For this review, take the finished solid that the model builds, in its own axes (mm). Coordinates: 2 decimals unless noted, no trailing zeros. Loops run counter-clockwise (first coordinate to the right, second up) from the corner with the lowest first, then second, coordinate; pieces in that order, holes last.
1. Take a section at B-B, the plane y = 2.2. Count the separate pieces of the cut face and the enclosed holes in it, then the cut area to 3 significant figures.
2. Take a section at C-C, the plane x = 0. State the section outline as (y, z) points.
3. Clearance check with flat-ended pins moving along their axes: P1, Ø3, axis at y = 4.5, z = -13, coming from the +X side; P2, Ø1, axis at y = 4, z = -2.5, coming from the +X side. State where each tip first meets the part, or that it passes through.
4. Mouldability with a two-part tool opening along Z and no side actions: class faces 1 (the face through (195.482, 2.535, -17.871)), 2 (the face through (-195.871, 2.535, 17.482)), 3 (the face through (-179.045, 2.465, -1.409)) as pulls with the +Z half, pulls with the -Z half, needs draft (parallel to the pull), parting line crosses it, or undercut.
5. To check wall thickness, follow probe 1 along X at (y, z) = (1, 0); probe 2 along Z at (x, y) = (163, 0.35); probe 3 along X at (y, z) = (2.05, -9.5). State the ranges of each line that lie inside material, in increasing order.
6. Take a section at A-A, the plane x = 172.7. State the section outline as (y, z) points.
```python
from build123d import *

# Parameters (mm, degrees)
SKETCH_1_W      = 406
SKETCH_1_H      = 50
SKETCH_1_R      = 6.5
SKETCH_1_R_2    = 9
SKETCH_1_R_3    = 2
EXTRUDE_1_DEPTH = 5
FILLET_1_R      = 25


with BuildPart() as part:
    # ｽｹｯﾁ1 → ﾎﾞｽ - 押し出し1 (new body)
    with BuildSketch(Plane(origin=(0, 0, 0), x_dir=(1, 0, 0), z_dir=(0, 1, 0))):
        Rectangle(SKETCH_1_W, SKETCH_1_H)
        with Locations(Location((172.7, 0, 0), (0, 0, 270))):
            Circle(SKETCH_1_R, mode=Mode.SUBTRACT)
        with Locations(Location((-172.7, 0, 0), (0, 0, 270))):
            Circle(SKETCH_1_R, mode=Mode.SUBTRACT)
        with Locations(Location((0, 0, 0), (0, 0, 270))):
            Circle(SKETCH_1_R_2, mode=Mode.SUBTRACT)
        with Locations(Location((12.02081528, 12.02081528, 0), (0, 0, 270))):
            Circle(SKETCH_1_R_3, mode=Mode.SUBTRACT)
        with Locations(Location((12.02081528, -12.02081528, 0), (0, 0, 270))):
            Circle(SKETCH_1_R_3, mode=Mode.SUBTRACT)
        with Locations(Location((-182.953048327, 10.253048327, 0), (0, 0, 270))):
            Circle(SKETCH_1_R_3, mode=Mode.SUBTRACT)
        with Locations(Location((182.953048327, 10.253048327, 0), (0, 0, 270))):
            Circle(SKETCH_1_R_3, mode=Mode.SUBTRACT)
        with Locations(Location((-182.953048327, -10.253048327, 0), (0, 0, 270))):
            Circle(SKETCH_1_R_3, mode=Mode.SUBTRACT)
        with Locations(Location((182.953048327, -10.253048327, 0), (0, 0, 270))):
            Circle(SKETCH_1_R_3, mode=Mode.SUBTRACT)
        with Locations(Location((-162.446951673, -10.253048327, 0), (0, 0, 270))):
            Circle(SKETCH_1_R_3, mode=Mode.SUBTRACT)
        with Locations(Location((-162.446951673, 10.253048327, 0), (0, 0, 270))):
            Circle(SKETCH_1_R_3, mode=Mode.SUBTRACT)
        with Locations(Location((-12.02081528, -12.02081528, 0), (0, 0, 270))):
            Circle(SKETCH_1_R_3, mode=Mode.SUBTRACT)
        with Locations(Location((162.446951673, -10.253048327, 0), (0, 0, 270))):
            Circle(SKETCH_1_R_3, mode=Mode.SUBTRACT)
        with Locations(Location((-12.02081528, 12.02081528, 0), (0, 0, 270))):
            Circle(SKETCH_1_R_3, mode=Mode.SUBTRACT)
        with Locations(Location((162.446951673, 10.253048327, 0), (0, 0, 270))):
            Circle(SKETCH_1_R_3, mode=Mode.SUBTRACT)
    extrude(amount=EXTRUDE_1_DEPTH)

    # ﾌｨﾚｯﾄ1
    fillet_1_edges = [part.edges().sort_by_distance(p)[0] for p in [
        (-203, 2.5, -25),
        (-203, 2.5, 25),
        (203, 2.5, 25),
        (203, 2.5, -25),
    ]]
    fillet(fillet_1_edges, radius=FILLET_1_R - 0.0001)  # a hair under: the kernel refuses the full size


solid = part.part
```
Results list:
1. separate pieces: 1
1. enclosed holes: 15
1. area: 19,100 mm2
2. outline: (0, -25) - (5, -25) - (5, -9) - (0, -9) - close; (0, 9) - (5, 9) - (5, 25) - (0, 25) - close
3. P1: stops at x = 200.2
3. P2: stops at x = 202.92
4. face 1: pulls with the -Z half
4. face 2: pulls with the +Z half
4. face 3: undercut
5. probe 1: x = -203 to -179.2, -166.2 to -9, 9 to 166.2, 179.2 to 203
5. probe 2: z = -25 to -12.18, -8.33 to 8.33, 12.18 to 25
5. probe 3: x = -201.12 to -184.81, -181.1 to -164.3, -160.59 to 160.59, 164.3 to 181.1, 184.81 to 201.12
6. outline: (0, -25) - (5, -25) - (5, -6.5) - (0, -6.5) - close; (0, 6.5) - (5, 6.5) - (5, 25) - (0, 25) - close
